from build123d import *

# Parameters (mm, degrees)
SALIENTE_EXTRUIR1_DEPTH = 1800
CROQUIS2_R              = 2.5
CORTAR_EXTRUIR1_DEPTH   = 1801.888669518
CROQUIS3_R              = 2.5
CORTAR_EXTRUIR2_DEPTH   = 10


with BuildPart() as part:
    # Croquis1 → Saliente-Extruir1 (new body)
    with BuildSketch(Plane.XY):
        Polygon((0, 0), (4, 0), (4, -36), (36, -36), (36, 0), (40, 0), (40, -40), (0, -40), align=None)
    extrude(amount=SALIENTE_EXTRUIR1_DEPTH)

    # Croquis2 → Cortar-Extruir1 (cut, through all)
    with BuildSketch(Plane.ZY):
        with Locations((9, -20)):
            Circle(CROQUIS2_R)
        with Locations((19, -20)):
            Circle(CROQUIS2_R)
    extrude(amount=-CORTAR_EXTRUIR1_DEPTH, mode=Mode.SUBTRACT)

    # Croquis3 → Cortar-Extruir2 (cut)
    with BuildSketch(Plane(origin=(0, -40, 0), x_dir=(-1, 0, 0), z_dir=(0, -1, 0))):
        with Locations(Location((-20, -9, 0), (0, 0, 180))):
            Circle(CROQUIS3_R)
        with Locations(Location((-20, -19, 0), (0, 0, 180))):
            Circle(CROQUIS3_R)
    extrude(amount=-CORTAR_EXTRUIR2_DEPTH, mode=Mode.SUBTRACT)


solid = part.part
Read the model definition and answer for the solid it produces. Units are mm, in the model's axes. A direction names the side the tool comes from. Coordinates: 2 decimals unless noted, no trailing zeros. Order: outer loops, then holes, each group sorted by start corner. A loop starts at its lowest first (then second) coordinate and runs counter-clockwise, first axis right, second up. Notation, with made-up numbers: (48.5, 57) - (75.5, 57) arc R13 cw to (75.5, 69) - close; hole circle Ø9 at (25, 76.25). An arc over 180 degrees is marked (long way). Use one line per item in the form item = value.
(1) Straight lines are drawn through the part: L1, parallel to Z at x = 20, y = -38.95; L2, parallel to X at y = -17, z = 1121.5; L3, parallel to Y at x = 2, z = 9. For each, find the intervals that lie inside material, in ascending order.
Computed values:
L1 = 0 to 6.5, 11.5 to 16.5, 21.5 to 1800
L2 = 0 to 4, 36 to 40
L3 = -40 to -22.5, -17.5 to 0
(2) For a pull along X with two mould halves and no side action, classify faces 3 (the face through (0, -20, 887)), 4 (the face through (20, -40, 887)), 5 (the face through (36, -18, 887)) as pulls with the +X half, pulls with the -X half, needs draft (parallel to the pull), parting line crosses it, or undercut.
Computed values:
face_3 = pulls with the -X half
face_4 = needs draft
face_5 = undercut
(3) Which of the six approach directions +Z, -Z, +X, -X, +Y, -Y give full straight-line access (tool end or side, diameter ignored) to faces 1 (the face through (20.1, -36.2, 1800)), 2 (the face through (20, -36, 887))?
Computed values:
face_1 = +Z, +X, -X, +Y, -Y
face_2 = +Z, -Z, +Y
(4) Section B-B, the plane x = 11 is taken. Give the vertices of the cut face in (y, z), then the cut area to 3 significant figures.
Computed values:
outline = (-40, 0) - (-36, 0) - (-36, 1800) - (-40, 1800) - close
area = 7,200 mm²
(5) Section A-A, the plane z = 679 is taken. Give the vertices of the cut face in (x, y), then the cut area to 3 significant figures.
Computed values:
outline = (0, -40) - (40, -40) - (40, 0) - (36, 0) - (36, -36) - (4, -36) - (4, 0) - (0, 0) - close
area = 448 mm²
